Geometry: final body of the model. Coordinates: model frame, mm. Round coordinates to 2 decimals unless told otherwise and drop trailing zeros. Loops run counter-clockwise (first coordinate to the right, second up) from the corner with the lowest first, then second, coordinate; pieces in that order, holes last. Notation, with made-up numbers: M 47,0 L 88,0 A26 ccw 88,15 Z; hole C 64.5,86 d4. An arc over 180 degrees is marked long. Answer as a JSON object with one key per item and string values.
from build123d import *

# Parameters (mm, degrees)
SKETCH1_W           = 393.7
SKETCH1_H           = 444.5
BOSS_EXTRUDE1_DEPTH = 3.175
CUT_EXTRUDE1_DEPTH  = 10


with BuildPart() as part:
    # Sketch1 → Boss-Extrude1 (new body)
    with BuildSketch(Plane(origin=(0, 0, 0), x_dir=(1, 0, 0), z_dir=(0, 1, 0))):
        Rectangle(SKETCH1_W, SKETCH1_H)
    extrude(amount=BOSS_EXTRUDE1_DEPTH)

    # Sketch2 → Cut-Extrude1 (cut)
    with BuildSketch(Plane(origin=(0, 3.175, 0), x_dir=(1, 0, 0), z_dir=(0, 1, 0))):
        with BuildLine():
            Line((-196.85, 222.25), (-156.718, 222.25))
            Line((-156.718, 222.25), (-156.718, 172.593))
            ThreePointArc((-156.718, 172.593), (-157.64793597, 170.34793597), (-159.893, 169.418))
            Line((-159.893, 169.418), (-196.85, 169.418))
            Line((-196.85, 169.418), (-196.85, 222.25))
        make_face()
        with BuildLine():
            Line((196.85, 222.25), (156.718, 222.25))
            Line((156.718, 222.25), (156.718, 172.593))
            ThreePointArc((156.718, 172.593), (157.64793597, 170.34793597), (159.893, 169.418))
            Line((159.893, 169.418), (196.85, 169.418))
            Line((196.85, 169.418), (196.85, 222.25))
        make_face()
    extrude(amount=-CUT_EXTRUDE1_DEPTH, mode=Mode.SUBTRACT)


solid = part.part
1) Section query A-A (y = 1). Return the cut outline in (x, z) (3 decimals), and give its area (3 significant figures).
Results:
{"outline": "M -196.85,-169.418 L -159.893,-169.418 A3.175 cw -156.718,-172.593 L -156.718,-222.25 L 156.718,-222.25 L 156.718,-172.593 A3.175 cw 159.893,-169.418 L 196.85,-169.418 L 196.85,222.25 L -196.85,222.25 Z", "area": "171,000 mm2"}
2) Ray query, line 1 (Z direction, x = -170, y = 2.35); line 2 (X direction, y = 2.75, z = -185.5). Return the intervals inside material, ascending.
Results:
{"line 1": "-169.42 to 222.25", "line 2": "-156.72 to 156.72"}
3) Pin query (flat end, axial travel): P1, Ø1, axis at x = -181, y = 1, coming from the -Z side; P2, Ø1.6, axis at y = 1, z = -191, coming from the +X side; P3, Ø1, axis at y = 1.5, z = -198, coming from the -X side. Return the tip coordinate at first contact, or that it passes through.
Results:
{"P1": "z = -169.42", "P2": "x = 156.72", "P3": "x = -156.72"}
4) Section query B-B (x = -171.5). Return the cut outline in (y, z) (3 decimals), and give its area (3 significant figures).
Results:
{"outline": "M 0,-169.418 L 3.175,-169.418 L 3.175,222.25 L 0,222.25 Z", "area": "1,240 mm2"}
5) Section query C-C (z = -180.5). Return the cut outline in (x, y) (3 decimals).
Results:
{"outline": "M -156.718,0 L 156.718,0 L 156.718,3.175 L -156.718,3.175 Z"}
